Could you check a few things on this model? Use its own coordinates, in mm. Face numbers are marked on the shaded views. A direction names the side the tool comes from. Coordinates: 2 decimals unless noted, no trailing zeros. Order: outer loops, then holes, each group sorted by start corner. A loop starts at its lowest first (then second) coordinate and runs counter-clockwise, first axis right, second up. Notation, with made-up numbers: (-34, -4.75) - (-27, -4.75) arc R12 cw to (-27, 7.25) - close; hole circle Ø4 at (76, 13). An arc over 180 degrees is marked (long way). One line per item, written item: value. Start each with the question number.
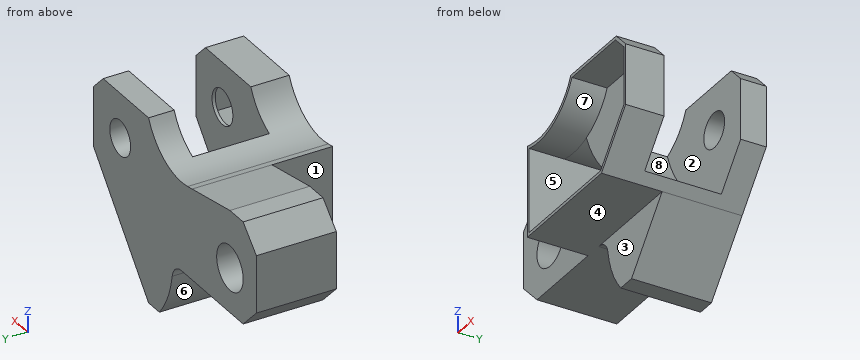
from build123d import *

# Parameters (mm, degrees)
F0_R     = 5.5
F0_R_2   = 7
F1_DEPTH = 44
F2_DEPTH = 19
F4_R     = 41
F5_DEPTH = 24
F7_DEPTH = 11
F9_DEPTH = 25


with BuildPart() as f1:
    # F0 (on Front) → F1 (new body)
    with BuildSketch(Plane.XZ):
        with BuildLine():
            Line((20, 14.47346), (20, -14))
            Line((20, -14), (25.575539, -14))
            Line((25.575539, -14), (59.205882, -14))
            Line((59.205882, -14), (72, 1))
            Line((72, 1), (72, 20))
            Line((72, 20), (67, 25))
            Line((67, 25), (43, 25))
            ThreePointArc((43, 25), (34.561099, 15.982044), (22.361381, 14.057085))
            Line((22.361381, 14.057085), (20, 14.47346))
        make_face()
        with Locations((58, 11)):
            Circle(F0_R, mode=Mode.SUBTRACT)
        Polygon((-14, 11), (-14, -7), (-7, -14), (20, -14), (20, 14.47346), (0, 18), (-7, 18), align=None)
        Circle(F0_R_2, mode=Mode.SUBTRACT)
        with BuildLine():
            Line((59.205882, -14), (25.575539, -14))
            ThreePointArc((25.575539, -14), (28.840775, -15.213414), (30.521178, -18.264706))
            ThreePointArc((30.521178, -18.264706), (32.858008, -26.115672), (37.29698, -33))
            Line((37.29698, -33), (43, -33))
            Line((43, -33), (59.205882, -14))
        make_face()
    extrude(amount=-F1_DEPTH)

    # F0 (on Front) → F2 (cut)
    with BuildSketch(Plane.XZ):
        Polygon((-14, 11), (-14, -7), (-7, -14), (20, -14), (20, 14.47346), (0, 18), (-7, 18), align=None)
        Circle(F0_R_2, mode=Mode.SUBTRACT)
        with BuildLine():
            Line((59.205882, -14), (25.575539, -14))
            ThreePointArc((25.575539, -14), (28.840775, -15.213414), (30.521178, -18.264706))
            ThreePointArc((30.521178, -18.264706), (32.858008, -26.115672), (37.29698, -33))
            Line((37.29698, -33), (43, -33))
            Line((43, -33), (59.205882, -14))
        make_face()
    extrude(amount=-F2_DEPTH, mode=Mode.SUBTRACT)

    # F4 (on offset) → F5 (cut)
    with BuildSketch(Plane.XZ.offset(-12)):
        with Locations((72, 28.701873)):
            Circle(F4_R)
    extrude(amount=-F5_DEPTH, mode=Mode.SUBTRACT)

    # F6 (on face) → F7 (cut)
    with BuildSketch(Plane.XZ):
        with BuildLine():
            ThreePointArc((43.636085, 24), (34.195381, 14.680891), (21, 13.319065))
            Line((21, 13.319065), (21, -13))
            Line((21, -13), (58.744476, -13))
            Line((58.744476, -13), (71, 1.368545))
            Line((71, 1.368545), (71, 19.585786))
            Line((71, 19.585786), (66.585786, 24))
            Line((66.585786, 24), (43.636085, 24))
        make_face()
    extrude(amount=-F7_DEPTH, mode=Mode.SUBTRACT)

    # F8 (on face) → F9 (cut, through all)
    with BuildSketch(Plane.XZ.offset(-11)):
        with BuildLine():
            Line((58.744476, -13), (59.986848, -11.543427))
            ThreePointArc((59.986848, -11.543427), (43.310182, -1.972127), (32.646683, 14.028209))
            ThreePointArc((32.646683, 14.028209), (26.876207, 12.805403), (21, 13.319065))
            Line((21, 13.319065), (21, -13))
            Line((21, -13), (58.744476, -13))
        make_face()
    extrude(amount=-F9_DEPTH, mode=Mode.SUBTRACT)


solid = f1.part
Q1. If I drill on L1, parallel to Z at x = 56, y = 7; L2, parallel to Z at x = 0, y = 25.25; L3, parallel to Y at x = -7.5, z = -2, over which ranges is the centre line in solid material (lowest first)?
Q2. We'd pull the mould along X, two halves only. Please class the marked faces 6, 7 and 8: +X half, -X half, draft (parallel to the pull), parting line (faces both ways), or undercut.
Q3. I want a section at B-B on z = 0. Please give me the cut outline in (x, y).
Q4. I want a section at A-A on y = 35. Please give me the cut outline in (x, z).
Q5. I want a section at D-D on y = 3. Please give me the cut outline in (x, z), then the cut area to 3 significant figures.
Q6. Which directions (+Z, -Z, +X, -X, +Y, -Y) give clear straight access to the entire face, cutting with the end or side of a thin tool? Please do the marked faces 1, 2, 3, 4 and 5.
Q7. I'm going to push flat-ended pins straight in: pin 1 (3.5 mm diameter, centred on x = -5, y = 30, fed in from +Z); pin 2 (3 mm diameter, centred on x = 9, y = 19, fed in from +Z); pin 3 (3 mm diameter, centred on x = 9, z = -1.5, fed in from -Y). Where does each tip first touch, or does it pass through?
Q8. I want a section at C-C on x = 57.5. Please give me the cut outline in (y, z).
Values follow:
1. L1: z = -14 to -13, 24 to 25
1. L2: z = -14 to -7, 7 to 18
1. L3: y = 19 to 44
2. face 6: -X half
2. face 7: undercut
2. face 8: +X half
3. outline: (-14, 19) - (-7, 19) - (-7, 44) - (-14, 44) - close; (7, 19) - (20, 19) - (20, 0) - (21, 0) - (21, 36) - (41.34, 36) - (41.34, 11) - (69.83, 11) - (69.83, 0) - (71.15, 0) - (71.15, 12) - (42.72, 12) - (42.72, 36) - (71.15, 36) - (71.15, 44) - (7, 44) - close
4. outline: (-14, -7) - (-7, -14) - (25.58, -14) arc R5 cw to (30.52, -18.26) arc R29 ccw to (37.3, -33) - (43, -33) - (61.76, -11) arc R41 cw to (33.24, 15.34) arc R19 cw to (22.36, 14.06) - (0, 18) - (-7, 18) - (-14, 11) - close; hole circle Ø14 at (0, 0); hole (21, -13) - (58.74, -13) - (59.99, -11.54) arc R42 cw to (32.65, 14.03) arc R20 cw to (21, 13.32) - close
5. outline: (20, -14) - (59.21, -14) - (72, 1) - (72, 20) - (67, 25) - (43, 25) arc R19 cw to (22.36, 14.06) - (20, 14.47) - close; hole (21, -13) - (58.74, -13) - (71, 1.37) - (71, 19.59) - (66.59, 24) - (43.64, 24) arc R20 cw to (21, 13.32) - close
5. area: 161 mm^2
6. face 1: +Z, -Z, -X, -Y
6. face 2: +Z, +X
6. face 3: -Z, +X, -X, -Y
6. face 4: -Z, -X, -Y
6. face 5: -Y
7. pin 1: stops at z = 18
7. pin 2: stops at z = 16.68
7. pin 3: stops at y = 19
8. outline: (0, -14) - (19, -14) - (19, -16) - (44, -16) - (44, 5.52) - (36, 5.52) - (36, -9.65) - (12, -9.65) - (12, 5.52) - (11, 5.52) - (11, -10.72) - (36, -10.72) - (36, -13) - (0, -13) - close; (0, 24) - (11, 24) - (11, 16.48) - (12, 16.48) - (12, 25) - (0, 25) - close; (36, 16.48) - (44, 16.48) - (44, 25) - (36, 25) - close
